Autodesk Inventor part; units mm, degrees
ref_plane "YZ Plane" through (0, 0, 0) normal (1, 0, 0) x (0, 1, 0)
ref_plane "XZ Plane" through (0, 0, 0) normal (0, 1, 0) x (-1, 0, 0)
ref_plane "XY Plane" through (0, 0, 0) normal (0, 0, 1) x (1, 0, 0)
sketch "Skizze1" plane through (0, 0, 0) normal (0, 0, 1) x (1, 0, 0)
  line L0 (-86.35, 2) -> (86.35, 2)
  line L1 (86.35, 2) -> (86.35, -2)
  line L2 (86.35, -2) -> (-86.35, -2)
  line L3 (-86.35, -2) -> (-86.35, 2)
  line L4 (-86.35, 2) -> (86.35, -2) construction
  line L5 (86.35, 2) -> (-86.35, -2) construction
  point P0 (0, 0)
  dimension "d0" = 4
  dimension "d1" = 172.7
extrude "Extrusion1" add sketch "Skizze1" along normal blind 172.7
sketch "Skizze2" plane through (-86.35, -2, 0) normal (0, -1, 0) x (1, 0, 0)
  line L0 (172.7, 0) -> (172.7, 172.7)
  line L1 (46.35, 136.35) -> (126.35, 136.35)
  line L2 (136.35, 126.35) -> (136.35, 46.35)
  line L3 (126.35, 36.35) -> (46.35, 36.35)
  line L4 (36.35, 46.35) -> (36.35, 126.35)
  line L5 (172.7, 0) -> (0, 0)
  line L6 (0, 0) -> (0, 172.7)
  line L7 (172.7, 172.7) -> (0, 172.7)
  arc A0 (46.35, 136.35) -> (36.35, 126.35) centre (46.35, 126.35) ccw
  arc A1 (36.35, 46.35) -> (46.35, 36.35) centre (46.35, 46.35) ccw
  arc A2 (126.35, 36.35) -> (136.35, 46.35) centre (126.35, 46.35) ccw
  arc A3 (136.35, 126.35) -> (126.35, 136.35) centre (126.35, 126.35) ccw
  point P0 (86.35, 0)
  point P1 (36.35, 136.35)
  point P2 (136.35, 136.35)
  point P3 (36.35, 36.35)
  dimension "d50" = 100
  dimension "d51" = 100
  dimension "d52" = 36.35
  dimension "d53" = 36.35
  dimension "d54" = 36.35
  dimension "d55" = 36.35
  dimension "d56" = 10
extrude "Extrusion2" cut sketch "Skizze2" against normal blind 10 contours L1 A3 L2 A2 L3 A1 L4 A0
sketch "Skizze3" plane through (-86.35, 2, 0) normal (0, 1, 0) x (1, 0, 0)
  line L0 (114.5855, -0.5055) -> (156.5746, -0.5055) construction
  line L1 (156.5746, -0.5055) -> (156.5746, -42.4946) construction
  line L2 (156.5746, -42.4946) -> (114.5855, -42.4946) construction
  line L3 (114.5855, -42.4946) -> (114.5855, -0.5055) construction
  point P0 (86.35, 0)
  dimension "d1" = 172.7
sketch "Skizze4" plane through (-86.35, 2, 0) normal (0, 1, 0) x (1, 0, 0)
  line L0 (0, -172.7) -> (172.7, -172.7)
  line L1 (0, -172.7) -> (10, -172.7)
  line L2 (10, -172.7) -> (10, -162.7)
  line L3 (10, -162.7) -> (0, -162.7)
  line L4 (0, -162.7) -> (0, -172.7)
  line L5 (0, 0) -> (0, -172.7)
  line L6 (0, 0) -> (10, 0)
  line L7 (10, 0) -> (10, -10)
  line L8 (10, -10) -> (0, -10)
  line L9 (0, -10) -> (0, 0)
  line L10 (172.7, 0) -> (162.7, 0)
  line L11 (162.7, 0) -> (162.7, -10)
  line L12 (162.7, -10) -> (172.7, -10)
  line L13 (172.7, -10) -> (172.7, 0)
  line L14 (172.7, 0) -> (172.7, -172.7)
  line L15 (172.7, -172.7) -> (162.7, -172.7)
  line L16 (162.7, -172.7) -> (162.7, -162.7)
  line L17 (162.7, -162.7) -> (172.7, -162.7)
  line L18 (172.7, -162.7) -> (172.7, -172.7)
  line L19 (172.7, 0) -> (0, 0)
  point P0 (86.35, 0)
  point P1 (0, -10)
  dimension "d57" = 10
  dimension "d58" = 10
  dimension "d59" = 10
  dimension "d60" = 10
  dimension "d61" = 10
  dimension "d62" = 10
  dimension "d63" = 10
extrude "Extrusion3" cut sketch "Skizze4" against normal blind 10 contours L4 L3 L2 L0 | L16 L17 L14 L0 | L5 L6 L7 L8 | L12 L11 L10 L13
fillet "Rundung1" radius 4 4 edges at (76.35, 0, 162.7) (76.35, 0, 10) (-76.35, 0, 10) (-76.35, 0, 162.7)
properties part number "Schutzglas_oben" material "Glas"
Could you check a few things on this model? Use its own coordinates, in mm. A direction names the side the tool comes from. Round coordinates to 2 decimals unless told otherwise and drop trailing zeros. Order: outer loops, then holes, each group sorted by start corner. A loop starts at its lowest first (then second) coordinate and runs counter-clockwise, first axis right, second up.
(1) Which directions (+Z, -Z, +X, -X, +Y, -Y) give clear straight access to the entire face, cutting with the end or side of a thin tool? Please do faces 4 (the flat face through (-76.35, 0, 3)), 5 (the flat face through (76.35, 0, 170)), 6 (the flat face through (-1, 0, 136.35)).
Response values:
face 4: -Z, -X, +Y, -Y
face 5: +Z, +X, +Y, -Y
face 6: +Y, -Y
(2) I'm going to push flat-ended pins straight in: pin 1 (1.2 mm diameter, centred on x = -84.5, y = -0.5, fed in from -Z); pin 2 (2 mm diameter, centred on y = 0.5, z = 171, fed in from -X); pin 3 (2 mm diameter, centred on x = -84.5, y = 0, fed in from +Z). Where does each tip first touch, or does it pass through?
Response values:
pin 1: stops at z = 10
pin 2: stops at x = -76.35
pin 3: stops at z = 162.7
(3) Imagine slicing it at C-C (y = -0.1). Write out the boundary of the cut face in (x, z).
Response values:
outline: (-86.35, 10) - (-80.35, 10) arc R4 cw to (-76.35, 6) - (-76.35, 0) - (76.35, 0) - (76.35, 6) arc R4 cw to (80.35, 10) - (86.35, 10) - (86.35, 162.7) - (80.35, 162.7) arc R4 cw to (76.35, 166.7) - (76.35, 172.7) - (-76.35, 172.7) - (-76.35, 166.7) arc R4 cw to (-80.35, 162.7) - (-86.35, 162.7) - close; hole (-50, 46.35) arc R10 ccw to (-40, 36.35) - (40, 36.35) arc R10 ccw to (50, 46.35) - (50, 126.35) arc R10 ccw to (40, 136.35) - (-40, 136.35) arc R10 ccw to (-50, 126.35) - close
(4) Please list where these lines run through material, in increasing order: line 1 along X through (y, z) = (-0.2, 79); line 2 along Z through (x, y) = (8, 1.8); line 3 along Z through (x, y) = (-41.5, -0.1).
Response values:
line 1: x = -86.35 to -50, 50 to 86.35
line 2: z = 0 to 36.35, 136.35 to 172.7
line 3: z = 0 to 36.46, 136.24 to 172.7
(5) Imagine slicing it at A-A (x = 21). Write out the boundary of the cut face in (y, z), plus the area to 3 significant figures.
Response values:
outline: (-2, 0) - (2, 0) - (2, 36.35) - (-2, 36.35) - close; (-2, 136.35) - (2, 136.35) - (2, 172.7) - (-2, 172.7) - close
area: 291 mm2
(6) Imagine slicing it at B-B (z = 66.5). Write out the boundary of the cut face in (x, y), plus the area to 3 significant figures.
Response values:
outline: (-86.35, -2) - (-50, -2) - (-50, 2) - (-86.35, 2) - close; (50, -2) - (86.35, -2) - (86.35, 2) - (50, 2) - close
area: 291 mm2
(7) If we mould it in two halves opening along X, with no side actions, what happens to faces 1 (the cylindrical face through (46.99, -0.03, 39.2)), 2 (the flat face through (-76.35, 0, 170)), 3 (the flat face through (83, 0, 162.7))? For each: released by +X, released by -X, zero draft, split by the parting line, or undercut.
Response values:
face 1: undercut
face 2: released by -X
face 3: zero draft
